Input: part model. Units: mm. Frame: model coordinates. A direction names the side the tool comes from. Coordinates: 2 decimals unless noted, no trailing zeros. Loops run counter-clockwise (first coordinate to the right, second up) from the corner with the lowest first, then second, coordinate; pieces in that order, holes last.
```python
from build123d import *

# Parameters (mm, degrees)
F0_R     = 17.272
F0_R_2   = 11.43
F1_DEPTH = 1.27
F2_R     = 12.573
F2_R_2   = 11.43
F3_DEPTH = 11.811
F5_DEPTH = 17.273
F7_DEPTH = 12.7
F9_DEPTH = 9.525


with BuildPart() as f1:
    # F0 (on Top) → F1 (new body)
    with BuildSketch(Plane.XY):
        Circle(F0_R)
        Circle(F0_R_2, mode=Mode.SUBTRACT)
    extrude(amount=F1_DEPTH)

    # F2 (on face) → F3 (join)
    with BuildSketch(Plane.XY.offset(1.27)):
        Circle(F2_R)
        Circle(F2_R_2, mode=Mode.SUBTRACT)
    extrude(amount=F3_DEPTH)

    # F4 (on Front) → F5 (cut, through all)
    with BuildSketch(Plane.XZ):
        with BuildLine():
            Line((-2.888614, 6.35), (2.888614, 6.35))
            ThreePointArc((2.888614, 6.35), (4.900767, 6.765492), (6.583774, 7.944))
            Line((6.583774, 7.944), (11.43, 13.081))
            Line((11.43, 13.081), (-11.43, 13.081))
            Line((-11.43, 13.081), (-6.583774, 7.944))
            ThreePointArc((-6.583774, 7.944), (-4.900767, 6.765492), (-2.888614, 6.35))
        make_face()
    extrude(amount=-F5_DEPTH, mode=Mode.SUBTRACT)

    # F6 (on Right) → F7 (cut, symmetric)
    with BuildSketch(Plane.YZ):
        Polygon((-12.573, 5.715), (5.237884, 13.081), (-12.573, 13.081), align=None)
    extrude(amount=F7_DEPTH, both=True, mode=Mode.SUBTRACT)

    # F8 (on face) → F9 (join)
    with BuildSketch(Plane.XY.offset(1.27)):
        with BuildLine():
            Line((2.193636, -14.310851), (1.905, -12.427844))
            ThreePointArc((1.905, -12.427844), (0, -12.573), (-1.905, -12.427844))
            Line((-1.905, -12.427844), (-2.193636, -14.310851))
            ThreePointArc((-2.193636, -14.310851), (0, -14.478), (2.193636, -14.310851))
        make_face()
    extrude(amount=F9_DEPTH)


solid = f1.part
```
Item 1: Reachability of faces 5 (the face through (-2.047, -13.356, 5.966)), 6 (the face through (0, 12, 6.35)), 7 (the face through (0.53, 12.56, 5.78)) from +Z, -Z, +X, -X, +Y, -Y: full face, straight path, thin tool, end or side. Return the list, or none.
Result:
face 5: +Z, -X
face 6: +Z, +Y
face 7: +Z
Item 2: Section query A-A (z = 3.5). Output: boundary loops of the cut face in (x, y) (3 decimals).
Result:
outline: (-2.194, -14.311) arc R14.478 ccw to (2.194, -14.311) - (1.905, -12.428) arc R12.573 ccw (long way) to (-1.905, -12.428) - close; hole circle Ø22.86 at (0, 0)
Item 3: Section query C-C (z = 9.75). Output: boundary loops of the cut face in (x, y) (1 decimal), then the cut area to 3 significant figures.
Result:
outline: (-12.3, -2.8) - (-11.1, -2.8) arc R11.4 cw to (-8.3, 7.9) - (-8.3, 9.5) arc R12.6 ccw to start; (-2.2, -14.3) arc R14.5 ccw to (2.2, -14.3) - (1.9, -12.4) arc R12.6 cw to (-1.9, -12.4) - close; (8.3, 7.9) arc R11.4 cw to (11.1, -2.8) - (12.3, -2.8) arc R12.6 ccw to (8.3, 9.5) - close
area: 36.5 mm2
Item 4: Mould query, pull axis X, two halves, no side actions, for faces 1 (the face through (0, -13, 10.795)), 2 (the face through (-9.198, 7.179, 10.715)), 3 (the face through (-0.031, -14.478, 5.966)), 4 (the face through (4.874, 10.77, 6.754)). Classes: +X half, -X half, draft (parallel to the pull), parting line (faces both ways), or undercut.
Result:
face 1: draft
face 2: undercut
face 3: parting line
face 4: undercut
Item 5: Section query B-B (y = 0). Output: boundary loops of the cut face in (x, z).
Result:
outline: (-17.27, 0) - (-11.43, 0) - (-11.43, 10.91) - (-12.57, 10.91) - (-12.57, 1.27) - (-17.27, 1.27) - close; (11.43, 0) - (17.27, 0) - (17.27, 1.27) - (12.57, 1.27) - (12.57, 10.91) - (11.43, 10.91) - close
Item 6: Contact query for flat-ended pins moving along their axis: P1, Ø2.5, axis at x = 0, y = -13, coming from the +Z side (3 decimals); P2, Ø5, axis at x = 6, z = 2, coming from the +Y side; P3, Ø4, axis at x = -2, y = 8, coming from the -Z side; P4, Ø3, axis at y = -11, z = 7, coming from the -X side. Output: stop coordinate, or through.
Result:
P1: stops at z = 10.795
P2: stops at y = 16.89
P3: passes through
P4: stops at x = -8.24
Item 7: Section query D-D (x = 0). Output: boundary loops of the cut face in (y, z) (3 decimals).
Result:
outline: (-17.272, 0) - (-11.43, 0) - (-11.43, 6.188) - (-12.573, 5.715) - (-12.573, 10.795) - (-14.478, 10.795) - (-14.478, 1.27) - (-17.272, 1.27) - close; (11.43, 0) - (17.272, 0) - (17.272, 1.27) - (12.573, 1.27) - (12.573, 6.35) - (11.43, 6.35) - close
Item 8: Line query: L1, parallel to Y at x = 0, z = 3; L2, parallel to X at y = 0, z = 9; L3, parallel to Z at x = 6, y = 15. Output: solid intervals per line, ascending.
Result:
L1: y = -14.48 to -11.43, 11.43 to 12.57
L2: x = -12.57 to -11.43, 11.43 to 12.57
L3: z = 0 to 1.27
